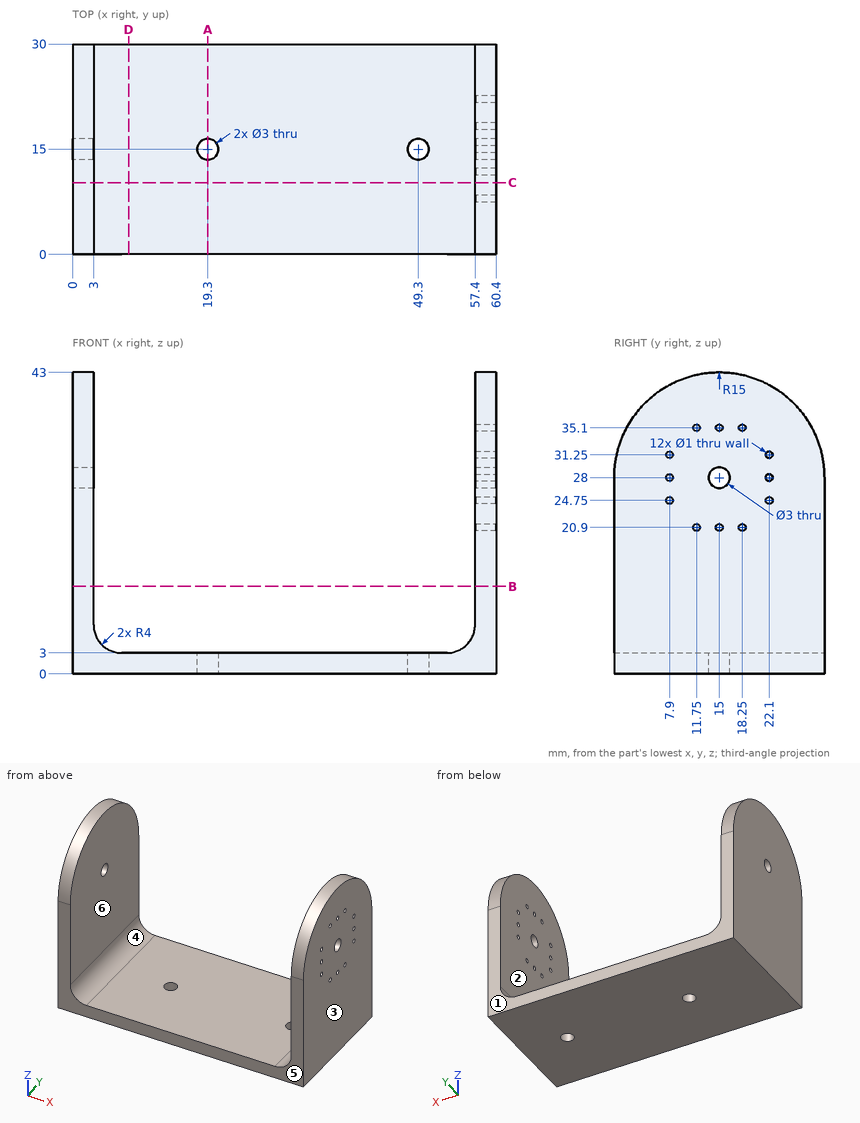
Verification items for this drawing (mm, ordinates from the low corner). A direction names the side the tool comes from. Coordinates: 2 decimals unless noted, no trailing zeros. Order: outer loops, then holes, each group sorted by start corner. A loop starts at its lowest first (then second) coordinate and runs counter-clockwise, first axis right, second up. Notation, with made-up numbers: (-2, 68) - (27, 68) arc R23 cw to (27, 82) - close; hole circle Ø7 at (0.25, 41.5). An arc over 180 degrees is marked (long way). Answer as a JSON object with one key per item and string values. Group by question number.
Item 1: Sectioned sample at D-D, the plane x = 8. Record the cut outline in (y, z).
Item 2: Sectioned sample at A-A, the plane x = 19.3. Record the cut outline in (y, z).
Item 3: Sectioned sample at B-B, the plane z = 12.5. Record the cut outline in (x, y).
Item 4: Tool access check on the marked faces 1 and 2. Record the directions out of +Z, -Z, +X, -X, +Y, -Y that give a thin tool (end or side, any length) a straight path to the whole face; none if there is none.
Item 5: Sectioned sample at C-C, the plane y = 10.25. Record the cut outline in (x, z), and give its area (3 significant figures).
Item 6: Scan lines: probe 1 along Y at (x, z) = (58.3, 20.9); probe 2 along X at (y, z) = (15, 1.85); probe 3 along X at (y, z) = (10.5, 39.5). Record each from-to range of solid material in increasing order.
Item 7: Depth check by flat-ended pin: pin 1 Ø5 at (y, z) = (15, 28) entering from +X; pin 2 Ø2.5 at (y, z) = (15, 28) entering from -X; pin 3 Ø9 at (x, y) = (31.5, 10) entering from +Z. Enter the tip coordinate at first touch or a pass-through.
Item 8: Draft check along X on the marked faces 3, 4, 5 and 6. Enter one of: +X half, -X half, draft (parallel to the pull), parting line (faces both ways), or undercut.
Resolved:
{
 "1": {"outline": "(0, 0) - (30, 0) - (30, 3) - (0, 3) - close"},
 "2": {"outline": "(0, 0) - (13.5, 0) - (13.5, 3) - (0, 3) - close; (16.5, 0) - (30, 0) - (30, 3) - (16.5, 3) - close"},
 "3": {"outline": "(0, 0) - (3, 0) - (3, 30) - (0, 30) - close; (57.4, 0) - (60.4, 0) - (60.4, 30) - (57.4, 30) - close"},
 "4": {"face 1": "+Z, -Z, +X, -X, +Y", "face 2": "+Z, +Y, -Y"},
 "5": {"outline": "(0, 0) - (60.4, 0) - (60.4, 42.23) - (57.4, 42.23) - (57.4, 7) arc R4 cw to (53.4, 3) - (7, 3) arc R4 cw to (3, 7) - (3, 42.23) - (0, 42.23) - close", "area": "423 mm^2"},
 "6": {"probe 1": "0 to 11.25, 12.25 to 14.5, 15.5 to 17.75, 18.75 to 30", "probe 2": "0 to 17.8, 20.8 to 47.8, 50.8 to 60.4", "probe 3": "0 to 3, 57.4 to 60.4"},
 "7": {"pin 1": "x = 60.4", "pin 2": "through", "pin 3": "z = 3"},
 "8": {"face 3": "+X half", "face 4": "undercut", "face 5": "draft", "face 6": "undercut"}
}
